from build123d import *

# Parameters (mm, degrees)
CROQUIS1_R              = 7.5
CROQUIS1_R_2            = 4
SALIENTE_EXTRUIR1_DEPTH = 24
CROQUIS2_W              = 2
CROQUIS2_H              = 1.8
CORTAR_EXTRUIR1_DEPTH   = 27.239283527
CROQUIS3_W              = 1
CROQUIS3_H              = 1


with BuildPart() as part:
    # Croquis1 → Saliente-Extruir1 (new body)
    with BuildSketch(Plane(origin=(0, 0, 0), x_dir=(1, 0, 0), z_dir=(0, 1, 0))):
        with Locations(Location((0, 0, 0), (0, 0, 270))):
            Circle(CROQUIS1_R)
        with Locations(Location((0, 0, 0), (0, 0, 270))):
            Circle(CROQUIS1_R_2, mode=Mode.SUBTRACT)
    extrude(amount=SALIENTE_EXTRUIR1_DEPTH)

    # Croquis2 → Cortar-Extruir1 (cut, through all)
    with BuildSketch(Plane.XZ):
        with Locations((7.445804188, 0)):
            Rectangle(CROQUIS2_W, CROQUIS2_H)
    extrude(amount=-CORTAR_EXTRUIR1_DEPTH, mode=Mode.SUBTRACT)

    # Cortar-Barrer3: sweep along a curve in space
    with BuildLine() as cortar_barrer3_path:
        ThreePointArc((0, 24, 4), (2.828427125, 24, 2.828427125), (4, 24, 0))
        ThreePointArc((4, 24, 0), (2.828427125, 24, -2.828427125), (0, 24, -4))
        ThreePointArc((0, 24, -4), (-2.828427125, 24, -2.828427125), (-4, 24, 0))
        ThreePointArc((-4, 24, 0), (-2.828427125, 24, 2.828427125), (0, 24, 4))
    # Croquis3 → Cortar-Barrer3 (sweep, cut)
    with BuildSketch(Plane.XY):
        with Locations((7.595804188, 20.25)):
            Rectangle(CROQUIS3_W, CROQUIS3_H)
        with Locations((7.595804188, 3.75)):
            Rectangle(CROQUIS3_W, CROQUIS3_H)
        with Locations((-7.595804188, 3.75)):
            Rectangle(CROQUIS3_W, CROQUIS3_H)
        with Locations((-7.595804188, 20.25)):
            Rectangle(CROQUIS3_W, CROQUIS3_H)
    sweep(path=cortar_barrer3_path.line, mode=Mode.SUBTRACT)


solid = part.part
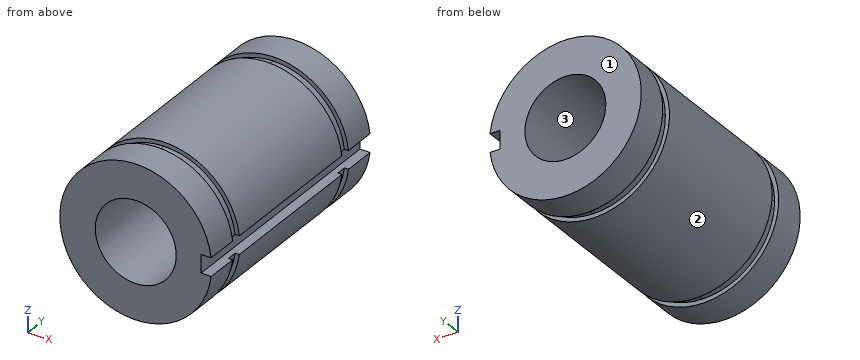
Could you check a few things on this model? Use its own coordinates, in mm. Face numbers are marked on the shaded views. Give positions to 0.01 mm unless a question says otherwise; leave off trailing zeros. Write each loop counter-clockwise with the first axis right and the second up, starting at its lowest first coordinate (ties: lowest second). Pieces come first, ordered by that corner, then holes. Notation, with made-up numbers: (41, 85.5) - (56, 85.5) arc R13 ccw to (56, 106.5) - close; hole circle Ø9 at (52, 27.25). An arc over 180 degrees is marked (long way). Use CSV: the item, a comma, the result in double quotes. Start each with the question number.
Item 1: If we mould it in two halves opening along X, with no side actions, what happens to the marked faces 1, 2 and 3? For each: pulls with the +X half, pulls with the -X half, needs draft (parallel to the pull), parting line crosses it, or undercut.
Item 2: I'm going to push flat-ended pins straight in: pin 1 (1.5 mm diameter, centred on y = 14.5, z = -6, fed in from +X); pin 2 (6.5 mm diameter, centred on x = 0, z = 0, fed in from -Y); pin 3 (3 mm diameter, centred on y = 15, z = 4, fed in from +X); pin 4 (0.8 mm diameter, centred on x = 7, y = 16.5, fed in from -Z). Where does each tip first touch, or does it pass through?
Item 3: I want a section at B-B, the plane y = 6.5. Please give me the cut outline in (x, z).
Item 4: I want a section at D-D, the plane x = -5.5. Please give me the cut outline in (y, z), then the cut area to 3 significant figures.
Item 5: If I drill on line 1 along X through (y, z) = (13.25, 0); line 2 along Z through (x, y) = (1, 1.75); line 3 along Z through (x, y) = (0.75, 8.5), over which ranges is the centre line in solid material (lowest first)?
Item 6: I want a section at A-A, the plane x = 1.75. Please give me the cut outline in (y, z).
Item 7: I want a section at C-C, the plane z = -5.25. Please give me the cut outline in (x, y), then the cut area to 3 significant figures.
Findings:
1,face 1,"needs draft"
1,face 2,"parting line crosses it"
1,face 3,"undercut"
2,pin 1,"stops at x = 5.36"
2,pin 2,"passes through"
2,pin 3,"stops at x = 7.07"
2,pin 4,"stops at z = -3.56"
3,outline,"(6.45, -0.9) - (6.45, 0.9) - (7.45, 0.9) arc R7.5 ccw (long way) to (7.45, -0.9) - close; hole circle Ø8 at (0, 0)"
4,outline,"(0, -5.1) - (3.25, -5.1) - (3.25, -4.48) - (4.25, -4.48) - (4.25, -5.1) - (19.75, -5.1) - (19.75, -4.48) - (20.75, -4.48) - (20.75, -5.1) - (24, -5.1) - (24, 5.1) - (20.75, 5.1) - (20.75, 4.48) - (19.75, 4.48) - (19.75, 5.1) - (4.25, 5.1) - (4.25, 4.48) - (3.25, 4.48) - (3.25, 5.1) - (0, 5.1) - close"
4,area,"242 mm2"
5,line 1,"x = -7.5 to -4, 4 to 6.45"
5,line 2,"z = -7.43 to -3.87, 3.87 to 7.43"
5,line 3,"z = -7.46 to -3.93, 3.93 to 7.46"
6,outline,"(0, -7.29) - (3.25, -7.29) - (3.25, -6.88) - (4.25, -6.88) - (4.25, -7.29) - (19.75, -7.29) - (19.75, -6.88) - (20.75, -6.88) - (20.75, -7.29) - (24, -7.29) - (24, -3.6) - (0, -3.6) - close; (0, 3.6) - (24, 3.6) - (24, 7.29) - (20.75, 7.29) - (20.75, 6.88) - (19.75, 6.88) - (19.75, 7.29) - (4.25, 7.29) - (4.25, 6.88) - (3.25, 6.88) - (3.25, 7.29) - (0, 7.29) - close"
7,outline,"(-5.36, 0) - (5.36, 0) - (5.36, 3.25) - (4.77, 3.25) - (4.77, 4.25) - (5.36, 4.25) - (5.36, 19.75) - (4.77, 19.75) - (4.77, 20.75) - (5.36, 20.75) - (5.36, 24) - (-5.36, 24) - (-5.36, 20.75) - (-4.77, 20.75) - (-4.77, 19.75) - (-5.36, 19.75) - (-5.36, 4.25) - (-4.77, 4.25) - (-4.77, 3.25) - (-5.36, 3.25) - close"
7,area,"255 mm2"
